```python
from build123d import *

# Parameters (mm, degrees)
SKETCH1_R           = 4
BOSS_EXTRUDE1_DEPTH = 15
SKETCH2_R           = 11.5
BOSS_EXTRUDE2_DEPTH = 5
SKETCH3_W           = 40
SKETCH3_H           = 58
BOSS_EXTRUDE3_DEPTH = 45
SKETCH6_R           = 15.5
BOSS_EXTRUDE4_DEPTH = 57
CHAMFER1_SIZE       = 0.5
FILLET1_R           = 1
SKETCH4_W           = 3.872983346
SKETCH4_H           = 7.5
CUT_EXTRUDE1_DEPTH  = 13


with BuildPart() as part:
    # Sketch1 → Boss-Extrude1 (new body)
    with BuildSketch(Plane(origin=(0, 0, 0), x_dir=(0, 0, -1), z_dir=(1, 0, 0))):
        Circle(SKETCH1_R)
    extrude(amount=BOSS_EXTRUDE1_DEPTH)

    # Sketch2 → Boss-Extrude2 (add)
    with BuildSketch(Plane.ZY):
        Circle(SKETCH2_R)
    extrude(amount=BOSS_EXTRUDE2_DEPTH)

    # Sketch3 → Boss-Extrude3 (add)
    with BuildSketch(Plane.ZY.offset(5)):
        with Locations((0, -6.5)):
            Rectangle(SKETCH3_W, SKETCH3_H)
    extrude(amount=BOSS_EXTRUDE3_DEPTH)

    # Sketch6 → Boss-Extrude4 (add)
    with BuildSketch(Plane.XZ.offset(35.5)):
        with Locations(Location((-27.5, 0, 0), (0, 0, 90))):
            Circle(SKETCH6_R)
    extrude(amount=BOSS_EXTRUDE4_DEPTH)

    # Chamfer1
    chamfer1_edges = [part.edges().sort_by_distance(p)[0] for p in [
        (15, 0, 4),
        (0, 0, -11.5),
    ]]
    chamfer(chamfer1_edges, length=CHAMFER1_SIZE)

    # Fillet1
    fillet1_edges = [part.edges().sort_by_distance(p)[0] for p in [
        (-27.5, 22.5, -20),
        (-5, -35.5, 0),
        (-27.5, -35.5, -20),
        (-5, -6.5, 20),
        (-27.5, -35.5, 20),
        (-5, 22.5, 0),
        (-27.5, 22.5, 20),
        (-50, -6.5, -20),
        (-50, -35.5, 0),
        (-50, -6.5, 20),
        (-50, 22.5, 0),
        (-27.5, -92.5, -15.5),
        (-5, -6.5, -20),
    ]]
    fillet(fillet1_edges, radius=FILLET1_R)

    # Sketch4 → Cut-Extrude1 (cut)
    with BuildSketch(Plane(origin=(15, 0, 0), x_dir=(0, 0, -1), z_dir=(1, 0, 0))):
        with Locations((0, 7.25)):
            Rectangle(SKETCH4_W, SKETCH4_H)
    extrude(amount=-CUT_EXTRUDE1_DEPTH, mode=Mode.SUBTRACT)


solid = part.part
```
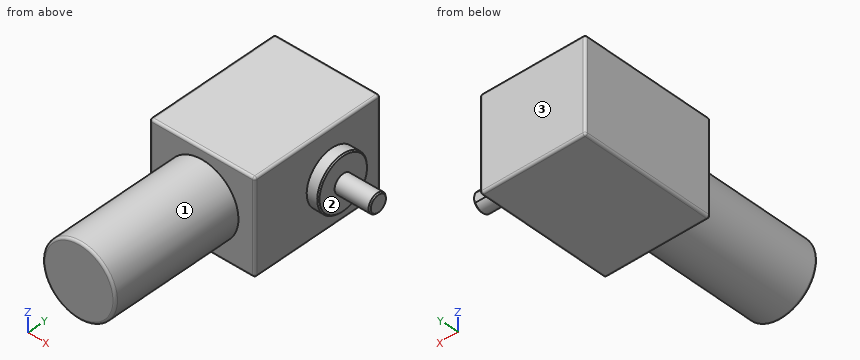
CAD build for the part. Positions are in the model's coordinates, mm. Face numbers are marked on the shaded views. A direction names the side the tool comes from. Coordinates: 2 decimals unless noted, no trailing zeros. Order: outer loops, then holes, each group sorted by start corner. A loop starts at its lowest first (then second) coordinate and runs counter-clockwise, first axis right, second up. Notation, with made-up numbers: (38, 82.25) - (92, 82.25) arc R14 ccw to (92, 89.25) - close; hole circle Ø6 at (0.5, 49). An arc over 180 degrees is marked (long way). Answer in a Markdown table with one row per item.
1. 3-axis set-ups, long thin cutter, end or side, ignore diameter. For the marked faces 1, 2 and 3: which of +Z, -Z, +X, -X, +Y, -Y reach the whole face in a straight line?
Answer:
| item | result |
|---|---|
| face 1 | -Y |
| face 2 | +X |
| face 3 | +Z, -Z, +X, -X, +Y |
2. Flat gauge pins, fed straight in: P1, Ø12, axis at x = -8, y = -64.5, coming from the +Z side; P2, Ø2, axis at x = -2.5, z = -6, coming from the -Y side; P3, Ø5, axis at x = -12.5, y = -70.5, coming from the -Z side; P4, Ø8, axis at x = -6.5, y = -56.5, coming from the -Z side. Where does each tip first touch, or does it go through?
Answer:
| item | result |
|---|---|
| P1 | z = 7.62 |
| P2 | y = -10.36 |
| P3 | z = -9.17 |
| P4 | through |
3. Drill centre lines: L1, parallel to X at y = -3, z = -12; L2, parallel to Y at x = -10.5, z = 15.5; L3, parallel to X at y = -77, z = 0. Where is each one in solid material? Low to high. Write a range as from..to.
Answer:
| item | result |
|---|---|
| L1 | -50..-5 |
| L2 | -35.5..22.5 |
| L3 | -43..-12 |
4. Slice it at B-B, the plane x = -9. List the corners of the cut face in (y, z).
Answer:
| item | result |
|---|---|
| outline | (-35.5, -19) arc R1 ccw to (-34.5, -20) - (21.5, -20) arc R1 ccw to (22.5, -19) - (22.5, 19) arc R1 ccw to (21.5, 20) - (-34.5, 20) arc R1 ccw to (-35.5, 19) - close |
5. Slice it at D-D, the plane y = -82.5. List the corners of the cut face in (x, z).
Answer:
| item | result |
|---|---|
| outline | circle Ø31 at (-27.5, 0) |
6. Slice it at A-A, the plane y = -13. List the corners of the cut face in (x, z).
Answer:
| item | result |
|---|---|
| outline | (-50, -19) arc R1 ccw to (-49, -20) - (-6, -20) arc R1 ccw to (-5, -19) - (-5, 19) arc R1 ccw to (-6, 20) - (-49, 20) arc R1 ccw to (-50, 19) - close |
7. Slice it at C-C, the plane x = -27.5. List the corners of the cut face in (y, z).
Answer:
| item | result |
|---|---|
| outline | (-92.5, -14.5) arc R1 ccw to (-91.5, -15.5) - (-35.5, -15.5) - (-35.5, -19) arc R1 ccw to (-34.5, -20) - (21.5, -20) arc R1 ccw to (22.5, -19) - (22.5, 19) arc R1 ccw to (21.5, 20) - (-34.5, 20) arc R1 ccw to (-35.5, 19) - (-35.5, 15.5) - (-91.5, 15.5) arc R1 ccw to (-92.5, 14.5) - close |
